```python
from build123d import *

# Parameters (mm, degrees)
BOSS_EXTRUDE1_DEPTH = 20
SKETCH2_W           = 24
SKETCH2_H           = 14
CUT_EXTRUDE1_DEPTH  = 24
SKETCH3_W           = 5
SKETCH3_H           = 12
CUT_EXTRUDE2_DEPTH  = 2
SKETCH4_W           = 2
SKETCH4_H           = 4
BOSS_EXTRUDE2_DEPTH = 4
CUT_EXTRUDE3_DEPTH  = 4


with BuildPart() as part:
    # Sketch1 → Boss-Extrude1 (new body)
    with BuildSketch(Plane(origin=(0, 0, 0), x_dir=(1, 0, 0), z_dir=(0, 1, 0))):
        Polygon((-28, 0), (0, 0), (0, 28), (-6, 28), (-6, 23), (-23, 6), (-28, 6), align=None)
    extrude(amount=BOSS_EXTRUDE1_DEPTH)

    # Sketch2 → Cut-Extrude1 (cut)
    with BuildSketch(Plane(origin=(0, 0, -28), x_dir=(-1, 0, 0), z_dir=(0, 0, -1))):
        with Locations((16, 10)):
            Rectangle(SKETCH2_W, SKETCH2_H)
    extrude(amount=-CUT_EXTRUDE1_DEPTH, mode=Mode.SUBTRACT)

    # Sketch3 → Cut-Extrude2 (cut)
    with BuildSketch(Plane.XY):
        with Locations((-23.25, 10)):
            Rectangle(SKETCH3_W, SKETCH3_H)
        with Locations((-4.75, 10)):
            Rectangle(SKETCH3_W, SKETCH3_H)
    cut_extrude2 = extrude(amount=-CUT_EXTRUDE2_DEPTH, mode=Mode.SUBTRACT)

    # Sketch4 → Boss-Extrude2 (add)
    with BuildSketch(Plane.XY.offset(-2)):
        with Locations((-24.75, 10)):
            Rectangle(SKETCH4_W, SKETCH4_H)
        with Locations((-3.25, 10)):
            Rectangle(SKETCH4_W, SKETCH4_H)
    boss_extrude2 = extrude(amount=BOSS_EXTRUDE2_DEPTH)

    # Mirror11: Cut-Extrude2, Boss-Extrude2 across plane
    add(cut_extrude2.mirror(Plane(origin=(0, 0, 0), x_dir=(0.707106781, 0, 0.707106781), z_dir=(-0.707106781, 0, 0.707106781))), mode=Mode.SUBTRACT)
    add(boss_extrude2.mirror(Plane(origin=(0, 0, 0), x_dir=(0.707106781, 0, 0.707106781), z_dir=(-0.707106781, 0, 0.707106781))))

    # Sketch5 → Cut-Extrude3 (cut)
    with BuildSketch(Plane(origin=(0, 0, -4), x_dir=(-1, 0, 0), z_dir=(0, 0, -1))):
        with BuildLine():
            Line((10.25, 12.5), (17.75, 12.5))
            ThreePointArc((17.75, 12.5), (20.25, 10), (17.75, 7.5))
            Line((17.75, 7.5), (10.25, 7.5))
            ThreePointArc((10.25, 7.5), (7.75, 10), (10.25, 12.5))
        make_face()
    cut_extrude3 = extrude(amount=-CUT_EXTRUDE3_DEPTH, mode=Mode.SUBTRACT)

    # Mirror12: Cut-Extrude3 across plane
    add(cut_extrude3.mirror(Plane(origin=(0, 0, 0), x_dir=(0.707106781, 0, 0.707106781), z_dir=(-0.707106781, 0, 0.707106781))), mode=Mode.SUBTRACT)


solid = part.part
```
The listing builds one solid part. Answer for the finished solid, in the listing's coordinates (mm). A direction names the side the tool comes from. Coordinates: 2 decimals unless noted, no trailing zeros. Write each loop counter-clockwise with the first axis right and the second up, starting at its lowest first coordinate (ties: lowest second). Pieces come first, ordered by that corner, then holes.
Q1. Given P1, Ø2, axis at x = 0.5, z = -24.5, coming from the -Y side; P2, Ø12, axis at y = 2.5, z = -9, coming from the +X side; P3, Ø6, axis at y = 13.5, z = -18.5, coming from the -X side; P4, Ø1.5, axis at x = -24.5, y = 2, coming from the -Z side, each flat-ended and moving along its own axis, determine where each tip first touches the part or whether it passes through.
Returned:
P1: stops at y = 0
P2: stops at x = 0
P3: stops at x = -4
P4: stops at z = -6
Q2. Section C-C, the plane x = -3 is taken. Write down the section's boundary in (y, z).
Returned:
outline: (0, -28) - (20, -28) - (20, 0) - (16, 0) - (16, -2) - (12, -2) - (12, 2) - (8, 2) - (8, -2) - (4, -2) - (4, 0) - (0, 0) - close; hole (7.5, -17.75) arc R2.5 ccw to (12.5, -17.75) - (12.5, -10.25) arc R2.5 ccw to (7.5, -10.25) - close
Q3. Section B-B, the plane y = 13 is taken. Write down the section's boundary in (x, z), then the cut area to 3 significant figures.
Returned:
outline: (-28, -4) - (-4, -4) - (-4, -28) - (0, -28) - (0, -25.75) - (-2, -25.75) - (-2, -20.75) - (0, -20.75) - (0, -7.25) - (-2, -7.25) - (-2, -2.25) - (0, -2.25) - (0, 0) - (-2.25, 0) - (-2.25, -2) - (-7.25, -2) - (-7.25, 0) - (-20.75, 0) - (-20.75, -2) - (-25.75, -2) - (-25.75, 0) - (-28, 0) - close
area: 168 mm2
Q4. Which of the six approach directions +Z, -Z, +X, -X, +Y, -Y give full straight-line access (tool end or side, diameter ignored) to faces 4 (the flat face through (-14, 7.5, -2)), 5 (the flat face through (-1, 16, -5)), 6 (the flat face through (-6, 1, -26)), 7 (the flat face through (-25, 12, 0)), 8 (the flat face through (-25.75, 10, 1))?
Returned:
face 4: +Z, -Z
face 5: +X
face 6: -Z, -X, +Y, -Y
face 7: +Z
face 8: +Z, -X, +Y, -Y
Q5. Find the intervals of material crossed by line 1 along Y through (x, z) = (-3.5, -1.25); line 2 along Y through (x, z) = (-1.5, -14.5); line 3 along Y through (x, z) = (-19, -5), in increasing order.
Returned:
line 1: y = 0 to 4, 8 to 12, 16 to 20
line 2: y = 0 to 7.5, 12.5 to 20
line 3: y = 0 to 3, 17 to 20
Q6. The mould has two halves that part along Z. Classify faces 1 (the flat face through (-2.25, 10, 1)), 2 (the flat face through (-14, 5, 0)), 3 (the flat face through (0, 10, -23.75)): released by +Z, released by -Z, zero draft, split by the parting line, or undercut.
Returned:
face 1: zero draft
face 2: released by +Z
face 3: undercut
Q7. Section A-A, the plane x = -11.5 is taken. Write down the section's boundary in (y, z).
Returned:
outline: (0, -17.5) - (3, -17.5) - (3, -4) - (7.5, -4) - (7.5, 0) - (0, 0) - close; (12.5, -4) - (17, -4) - (17, -17.5) - (20, -17.5) - (20, 0) - (12.5, 0) - close
Q8. Section D-D, the plane z = -24.5 is taken. Write down the section's boundary in (x, y), then the cut area to 3 significant figures.
Returned:
outline: (-6, 0) - (0, 0) - (0, 4) - (-2, 4) - (-2, 8) - (2, 8) - (2, 12) - (-2, 12) - (-2, 16) - (0, 16) - (0, 20) - (-6, 20) - (-6, 17) - (-4, 17) - (-4, 3) - (-6, 3) - close
area: 84.0 mm2
